Verification items for the finished model (mm, model axes). A direction names the side the tool comes from. Round coordinates to 2 decimals unless told otherwise and drop trailing zeros. Write each loop counter-clockwise with the first axis right and the second up, starting at its lowest first coordinate (ties: lowest second). Pieces come first, ordered by that corner, then holes. Notation, with made-up numbers: M 58.5,-19 L 109.5,-19 A16 cw 109.5,-9 Z; hole C -16.5,87.25 d7. An arc over 180 degrees is marked long. One line per item, written item: value. Start each with the question number.
Item 1: Gauge pin test, flat ends, axial feed: pin 1 (7 mm diameter, centred on x = 263.52, y = 26.03, fed in from -Z); pin 2 (2 mm diameter, centred on x = 226.5, y = 56.5, fed in from +Z); pin 3 (1.5 mm diameter, centred on x = 148.5, z = -4, fed in from -Y). Record the tip position at first contact, or that the pin passes through.
Item 2: Thickness scan on probe 1 along X at (y, z) = (53, -17.75); probe 2 along X at (y, z) = (104, -10.5); probe 3 along X at (y, z) = (37, -11). Record the ranges inside material, lowest first. Write a range as from..to.
Item 3: Section check B-B, the plane y = 226.5. Record the cut outline in (x, z), then the cut area to 3 significant figures.
Item 4: Tool access check on faces 1 (the face through (105.41, 74, -13)), 2 (the face through (38.1, 145, -16)), 3 (the face through (265.4, 261, -5)). Record the directions out of +Z, -Z, +X, -X, +Y, -Y that give a thin tool (end or side, any length) a straight path to the whole face; none if there is none.
Item 5: Draft check along X on faces 4 (the face through (29, 24, -5)), 5 (the face through (20.96, 151.12, -1.81)), 6 (the face through (145, 16.331, -13)). Enter one of: +X half, -X half, draft (parallel to the pull), parting line (faces both ways), or undercut.
Item 6: Section check A-A, the plane x = 159. Record the cut outline in (y, z).
from build123d import *

# Parameters (mm, degrees)
F1_DEPTH = 19.05
F0_R     = 4.25
F2_DEPTH = 12.7
F0_R_2   = 1.5875
F3_DEPTH = 5
F4_R     = 6.35


with BuildPart() as f1:
    # F0 (on Top) → F1 (new body)
    with BuildSketch(Plane.XY):
        with BuildLine():
            Line((38.1, 270.509999), (38.1, 16.509999))
            Line((38.1, 16.509999), (69.85, 16.509999))
            Line((69.85, 16.509999), (69.85, 129.294202))
            ThreePointArc((69.85, 129.294202), (87.629852, 147.074053), (105.409704, 129.294202))
            Line((105.409704, 129.294202), (105.409704, 16.33076))
            Line((105.409704, 16.33076), (186.690297, 16.33076))
            Line((186.690297, 16.33076), (186.690297, 129.294202))
            ThreePointArc((186.690297, 129.294202), (204.470149, 147.074053), (222.25, 129.294202))
            Line((222.25, 129.294202), (222.25, 16.509999))
            Line((222.25, 16.509999), (254, 16.509999))
            Line((254, 16.509999), (254, 270.509999))
            Line((254, 270.509999), (38.1, 270.509999))
        make_face()
    extrude(amount=-F1_DEPTH)

    # F0 (on Top) → F2 (join)
    with BuildSketch(Plane.XY):
        Polygon((19.05, 289.559999), (19.05, 16.509999), (38.1, 16.509999), (38.1, 270.509999), (254, 270.509999), (254, 16.509999), (273.05, 16.509999), (273.05, 289.559999), align=None)
        with Locations((28.575, 26.034999)):
            Circle(F0_R, mode=Mode.SUBTRACT)
        with Locations((28.574999, 104.351665)):
            Circle(F0_R, mode=Mode.SUBTRACT)
        with Locations((263.525, 26.034999)):
            Circle(F0_R, mode=Mode.SUBTRACT)
        with Locations((263.525001, 104.351665)):
            Circle(F0_R, mode=Mode.SUBTRACT)
        with Locations((28.574999, 182.668321)):
            Circle(F0_R, mode=Mode.SUBTRACT)
        with Locations((28.575, 260.984987)):
            Circle(F0_R, mode=Mode.SUBTRACT)
        with Locations((47.625, 280.034989)):
            Circle(F0_R, mode=Mode.SUBTRACT)
        with Locations((263.525001, 182.668321)):
            Circle(F0_R, mode=Mode.SUBTRACT)
        with Locations((146.05, 280.034989)):
            Circle(F0_R, mode=Mode.SUBTRACT)
        with Locations((263.525, 260.984987)):
            Circle(F0_R, mode=Mode.SUBTRACT)
        with Locations((244.475, 280.034989)):
            Circle(F0_R, mode=Mode.SUBTRACT)
    extrude(amount=-F2_DEPTH)

    # F0 (on Top) → F3 (join)
    with BuildSketch(Plane.XY):
        with Locations((263.525, 26.034999)):
            Circle(F0_R)
        with Locations((263.525, 26.034999)):
            Circle(F0_R_2, mode=Mode.SUBTRACT)
        with Locations((263.525001, 104.351665)):
            Circle(F0_R)
        with Locations((263.525001, 104.351665)):
            Circle(F0_R_2, mode=Mode.SUBTRACT)
        with Locations((263.525001, 182.668321)):
            Circle(F0_R)
        with Locations((263.525001, 182.668321)):
            Circle(F0_R_2, mode=Mode.SUBTRACT)
        with Locations((263.525, 260.984987)):
            Circle(F0_R)
        with Locations((263.525, 260.984987)):
            Circle(F0_R_2, mode=Mode.SUBTRACT)
        with Locations((244.475, 280.034989)):
            Circle(F0_R)
        with Locations((244.475, 280.034989)):
            Circle(F0_R_2, mode=Mode.SUBTRACT)
        with Locations((146.05, 280.034989)):
            Circle(F0_R)
        with Locations((146.05, 280.034989)):
            Circle(F0_R_2, mode=Mode.SUBTRACT)
        with Locations((47.625, 280.034989)):
            Circle(F0_R)
        with Locations((47.625, 280.034989)):
            Circle(F0_R_2, mode=Mode.SUBTRACT)
        with Locations((28.575, 260.984987)):
            Circle(F0_R)
        with Locations((28.575, 260.984987)):
            Circle(F0_R_2, mode=Mode.SUBTRACT)
        with Locations((28.574999, 182.668321)):
            Circle(F0_R)
        with Locations((28.574999, 182.668321)):
            Circle(F0_R_2, mode=Mode.SUBTRACT)
        with Locations((28.574999, 104.351665)):
            Circle(F0_R)
        with Locations((28.574999, 104.351665)):
            Circle(F0_R_2, mode=Mode.SUBTRACT)
        with Locations((28.575, 26.034999)):
            Circle(F0_R)
        with Locations((28.575, 26.034999)):
            Circle(F0_R_2, mode=Mode.SUBTRACT)
    extrude(amount=-F3_DEPTH)

    # F4
    f4_edges = [f1.edges().sort_by_distance(p)[0] for p in [
        (19.05, 153.034999, 0),
        (44.45, 16.509999, 0),
        (69.85, 72.9021, 0),
        (146.05, 16.33076, 0),
        (186.690297, 72.812481, 0),
        (247.65, 16.509999, 0),
        (273.05, 153.034999, 0),
    ]]
    fillet(f4_edges, radius=F4_R)


solid = f1.part
Response values:
1. pin 1: stops at z = -5
1. pin 2: stops at z = -0.1
1. pin 3: stops at y = 16.54
2. probe 1: x = 38.1..69.85, 105.41..186.69, 222.25..254
2. probe 2: x = 19.05..24.34, 32.81..69.85, 105.41..186.69, 222.25..259.29, 267.76..273.05
2. probe 3: x = 19.05..69.85, 105.41..186.69, 222.25..273.05
3. outline: M 19.05,-12.7 L 38.1,-12.7 L 38.1,-19.05 L 254,-19.05 L 254,-12.7 L 273.05,-12.7 L 273.05,-6.35 A6.35 ccw 266.7,0 L 25.4,0 A6.35 ccw 19.05,-6.35 Z
3. area: 4,580 mm2
4. face 1: +Z, -Z, -Y
4. face 2: -Z, -X, +Y, -Y
4. face 3: -Z
5. face 4: undercut
5. face 5: -X half
5. face 6: draft
6. outline: M 16.33,-19.05 L 270.51,-19.05 L 270.51,-12.7 L 289.56,-12.7 L 289.56,0 L 22.68,0 A6.35 ccw 16.33,-6.35 Z
